The drawing under review shows one solid part. Ordinate dimensions are in mm from its lowest x, y, z. A direction names the side the tool comes from. Coordinates: 2 decimals unless noted, no trailing zeros. Loops run counter-clockwise (first coordinate to the right, second up) from the corner with the lowest first, then second, coordinate; pieces in that order, holes last. Notation, with made-up numbers: M -32.5,43.25 L 7.5,43.25 A17 cw 7.5,68.25 Z; hole C -3.75,-13.5 d3. An arc over 180 degrees is marked long. Return JSON: item names as keys, results as strings.
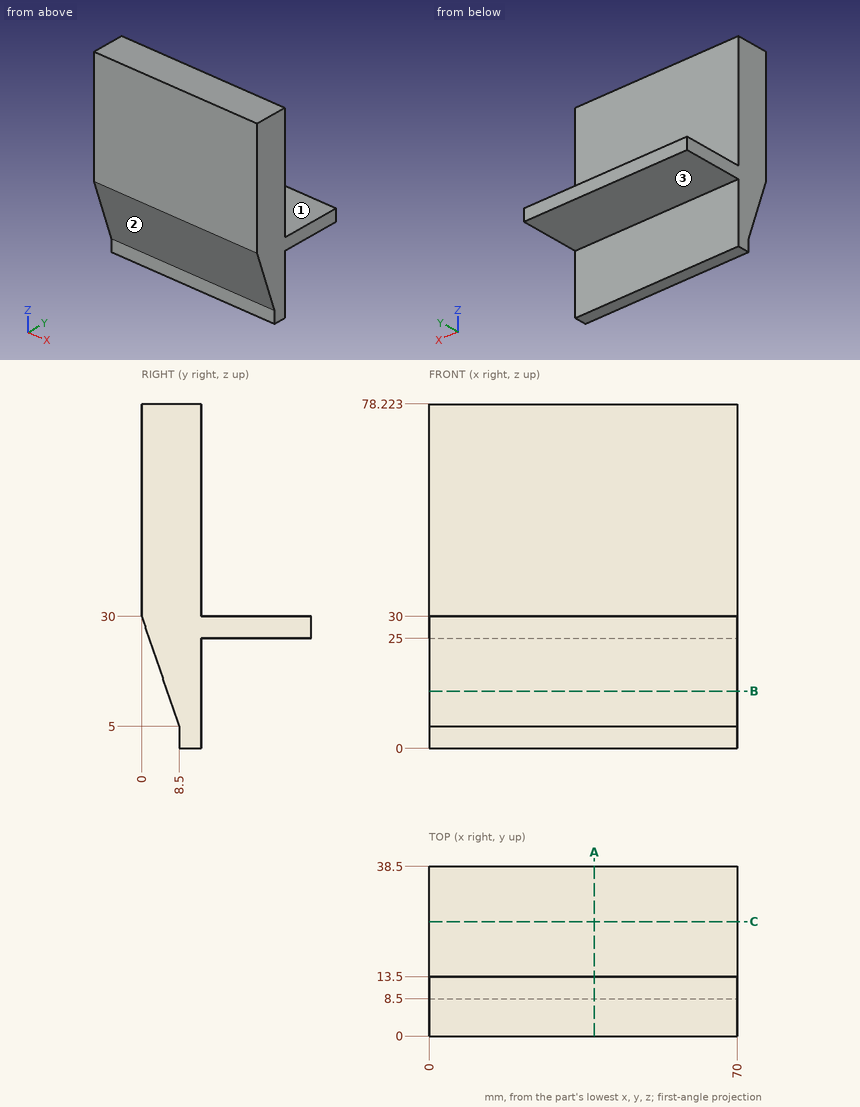
1. Add section B-B on z = 13. Give the boundary of the cut face in (x, y).
Check values:
{"outline": "M 0,5.78 L 70,5.78 L 70,13.5 L 0,13.5 Z"}
2. Add section A-A on x = 37.5. Give the boundary of the cut face in (y, z).
Check values:
{"outline": "M 0,30 L 8.5,5 L 8.5,0 L 13.5,0 L 13.5,25 L 38.5,25 L 38.5,30 L 13.5,30 L 13.5,78.22 L 0,78.22 Z"}
3. Machinability: for the marked faces 1, 2 and 3, which of the approach directions +Z, -Z, +X, -X, +Y, -Y give a long, thin tool a straight path to every point of the face, cutting with its end or side? Answer none if there is none.
Check values:
{"face 1": "+Z, +X, -X, +Y", "face 2": "-Z, +X, -X, -Y", "face 3": "-Z, +X, -X, +Y"}
4. To check wall thickness, follow line 1 (Z direction, x = 4, y = 21); line 2 (Y direction, x = 12, z = 39.5); line 3 (Y direction, x = 42, z = 17.5). State the ranges of each line that lie inside material, in increasing order.
Check values:
{"line 1": "25 to 30", "line 2": "0 to 13.5", "line 3": "4.25 to 13.5"}
5. Insertion check: pin 1 Ø5 at (x, z) = (42, 35) entering from +Y; pin 2 Ø10 at (x, z) = (23, 15.5) entering from -Y; pin 3 Ø3 at (x, z) = (42.5, 28) entering from -Y. Each pin has a flat end and moves straight along its axis. Give the tip position at first contact, or say it passes through.
Check values:
{"pin 1": "y = 13.5", "pin 2": "y = 3.23", "pin 3": "y = 0.17"}
6. Add section C-C on y = 26. Give the boundary of the cut face in (x, z).
Check values:
{"outline": "M 0,25 L 70,25 L 70,30 L 0,30 Z"}
